Answer from the drawing. Dimensions are ordinates in mm from the lowest x, y and z of the part. A direction names the side the tool comes from. Round coordinates to 2 decimals unless told otherwise and drop trailing zeros. Loops run counter-clockwise (first coordinate to the right, second up) from the corner with the lowest first, then second, coordinate; pieces in that order, holes last. Notation, with made-up numbers: (48.25, 61.25) - (93.25, 61.25) arc R18 ccw to (93.25, 76.25) - close; hole circle Ø8 at (-4, -2.5). An arc over 180 degrees is marked (long way). Answer as CSV lines item,"result".
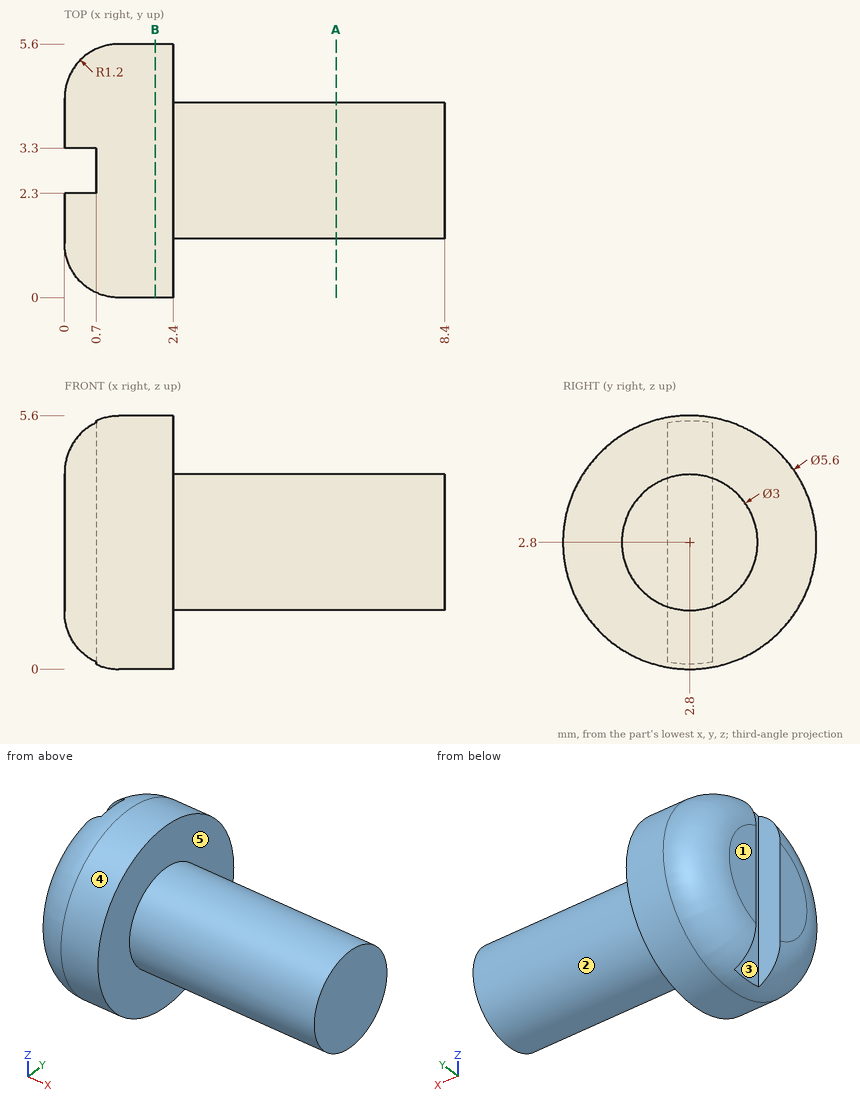
1) Find the intervals of material crossed by line 1 (X direction, y = 2.75, z = 2.6); line 2 (X direction, y = 2.65, z = 0.4); line 3 (Y direction, x = 5.5, z = 2.85), in increasing order.
Entries:
line 1,"x = 0.7 to 8.4"
line 2,"x = 0.7 to 2.4"
line 3,"y = 1.3 to 4.3"
2) A cutting plane is placed at A-A, the plane x = 6. Determine the outline of the cut face in (y, z), plus the area to 3 significant figures.
Entries:
outline,"circle Ø3 at (2.8, 2.8)"
area,"7.07 mm^2"
3) A tool of negligible diameter and unlimited length cuts with its end or side. For the marked faces 4 and 5, from which of +Z, -Z, +X, -X, +Y, -Y can it reach the whole face along a straight path? Write none if from no direction.
Entries:
face 4,"+X, -X"
face 5,"+X"
4) Each of these flat-tipped pins is pushed along its axis until it touches: P1, Ø3, axis at x = 7, z = 3, coming from the -Y side; P2, Ø1, axis at x = 3.5, y = 1, coming from the +Z side; P3, Ø3, axis at x = 5, z = 0.5, coming from the -Y side. Where does it stop, or does it pass through?
Entries:
P1,"stops at y = 1.3"
P2,"stops at z = 3.55"
P3,"stops at y = 1.53"
5) A cutting plane is placed at B-B, the plane x = 2. Determine the outline of the cut face in (y, z), plus the area to 3 significant figures.
Entries:
outline,"circle Ø5.6 at (2.8, 2.8)"
area,"24.6 mm^2"
6) The mould has two halves that part along Y. Classify the marked faces 1, 2 and 3: pulls with the +Y half, pulls with the -Y half, needs draft (parallel to the pull), parting line crosses it, or undercut.
Entries:
face 1,"needs draft"
face 2,"parting line crosses it"
face 3,"undercut"
